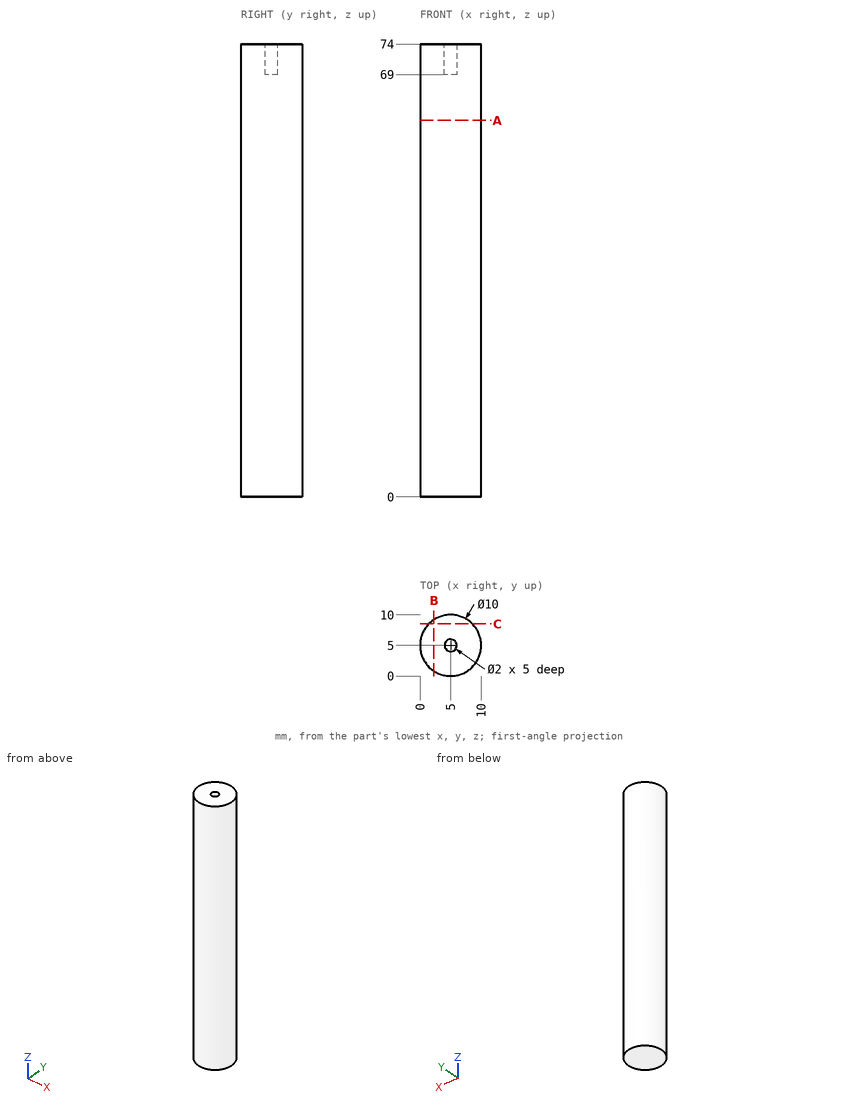
Source: three-view drawing plus pictorial views. Frame: mm from the lowest corner of the part. Round coordinates to 2 decimals unless told otherwise and drop trailing zeros. Loops run counter-clockwise (first coordinate to the right, second up) from the corner with the lowest first, then second, coordinate; pieces in that order, holes last.
Q1. Section A-A on z = 61.5. Return loops of the section in (x, y), plus the area to 3 significant figures.
Q2. Material intervals for L1, parallel to Y at x = 5, z = 71; L2, parallel to X at y = 2.75, z = 9.5; L3, parallel to Y at x = 1.25, z = 13, sorted ascending.
Q3. Pin query (flat end, axial travel): P1, Ø1, axis at y = 4, z = 49.5, coming from the +X side; P2, Ø2.5, axis at x = 5, y = 5, coming from the +Z side; P3, Ø3, axis at x = 9, z = 65, coming from the -Y side. Return the tip coordinate at first contact, or that it passes through.
Q4. Section C-C on y = 8.5. Return loops of the section in (x, z), plus the area to 3 significant figures.
Q5. Section B-B on x = 2.25. Return loops of the section in (y, z).
Evaluation:
1. outline: circle Ø10 at (5, 5)
1. area: 78.5 mm2
2. L1: y = 0 to 4, 6 to 10
2. L2: x = 0.53 to 9.47
2. L3: y = 1.69 to 8.31
3. P1: stops at x = 9.97
3. P2: stops at z = 74
3. P3: stops at y = 0.67
4. outline: (1.43, 0) - (8.57, 0) - (8.57, 74) - (1.43, 74) - close
4. area: 528 mm2
5. outline: (0.82, 0) - (9.18, 0) - (9.18, 74) - (0.82, 74) - close
